Geometry: see drawing. Coordinates: mm, zero at the bounding-box minimum. A direction names the side the tool comes from. Coordinates: 2 decimals unless noted, no trailing zeros. Order: outer loops, then holes, each group sorted by start corner. A loop starts at its lowest first (then second) coordinate and runs counter-clockwise, first axis right, second up. Notation, with made-up numbers: M -38.75,52 L -10.75,52 A23 ccw -10.75,88 Z; hole C 3.5,58.5 d11. An arc over 180 degrees is marked long. One line per item, written item: value.
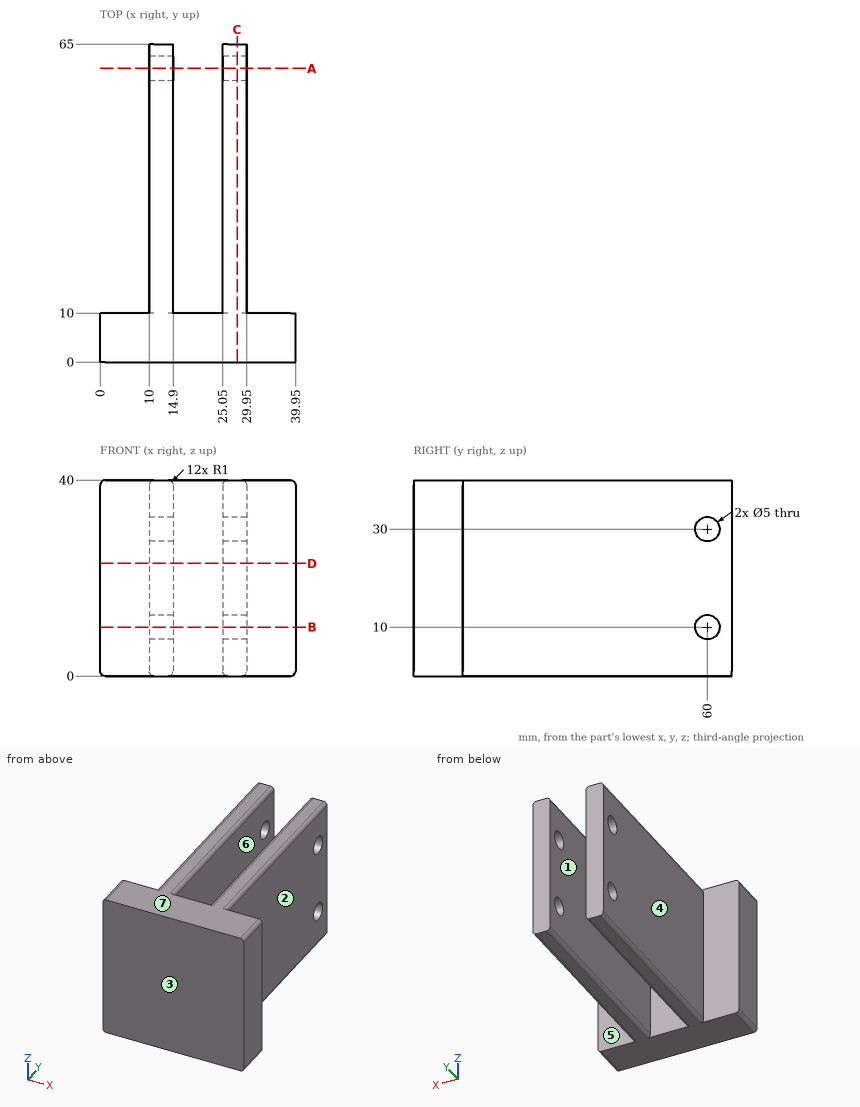
(1) Draft query along X for the marked faces 1, 2, 3 and 4. Return one class per face: released by +X, released by -X, zero draft, split by the parting line, or undercut.
Data:
face 1: undercut
face 2: released by +X
face 3: zero draft
face 4: released by -X
(2) Access query for the marked faces 5, 6 and 7. Directions: +Z, -Z, +X, -X, +Y, -Y. A direction counts if a zero-diameter tool reaches every point of the face in a straight line with its end or side. Return the directions, or none.
Data:
face 5: +Z, -Z, +X, +Y
face 6: +Z, -Z, +Y
face 7: +Z, +X, -X, +Y, -Y
(3) Cut plane C-C on x = 28. Output: boundary loops of the cut face in (y, z), plus the area to 3 significant figures.
Data:
outline: M 0,0 L 65,0 L 65,40 L 0,40 Z; hole C 60,10 d5; hole C 60,30 d5
area: 2,560 mm2
(4) Cut plane B-B on z = 10. Output: boundary loops of the cut face in (x, y).
Data:
outline: M 0,0 L 39.95,0 L 39.95,10 L 29.95,10 L 29.95,57.5 L 25.05,57.5 L 25.05,10 L 14.9,10 L 14.9,57.5 L 10,57.5 L 10,10 L 0,10 Z; M 10,62.5 L 14.9,62.5 L 14.9,65 L 10,65 Z; M 25.05,62.5 L 29.95,62.5 L 29.95,65 L 25.05,65 Z
(5) Ray query, line 1 (X direction, y = 45.5, z = 17.5); line 2 (Y direction, x = 29, z = 10); line 3 (Y direction, x = 17, z = 30). Return the intervals inside material, ascending. Write a range as from..to.
Data:
line 1: x = 10..14.9, 25.05..29.95
line 2: y = 0..57.5, 62.5..65
line 3: y = 0..10
(6) First-contact query: pin 1 (3 mm diameter, centred on y = 17.5, z = 6, fed in from +X); pin 2 (5 mm diameter, centred on x = 31.5, z = 27, fed in from +Y); pin 3 (5.5 mm diameter, centred on x = 4, z = 24.5, fed in from +Y); pin 4 (3 mm diameter, centred on y = 60, z = 10, fed in from +X). Flat tips, straight axial feed; report the tip coordinate or a pass-through.
Data:
pin 1: stops at x = 29.95
pin 2: stops at y = 65
pin 3: stops at y = 10
pin 4: passes through
(7) Cut plane A-A on y = 60. Give the number of separate pieces and of enclosed holes in the cut face, plus the area to 3 significant figures.
Data:
separate pieces: 6
enclosed holes: 0
area: 292 mm2
(8) Cut plane D-D on z = 23. Output: boundary loops of the cut face in (x, y), plus the area to 4 significant figures.
Data:
outline: M 0,0 L 39.95,0 L 39.95,10 L 29.95,10 L 29.95,65 L 25.05,65 L 25.05,10 L 14.9,10 L 14.9,65 L 10,65 L 10,10 L 0,10 Z
area: 938.5 mm2
